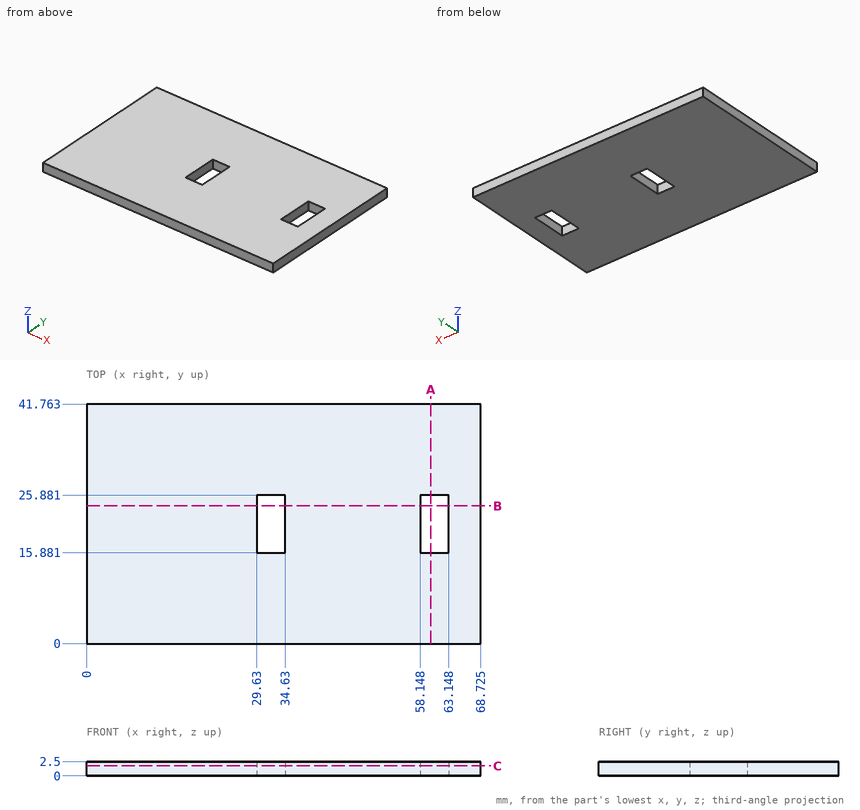
Job drawing, mm, ordinate dimensions from the low corner. One solid piece. Give positions to 0.01 mm unless a question says otherwise; leave off trailing zeros. Write each loop counter-clockwise with the first axis right and the second up, starting at its lowest first coordinate (ties: lowest second). Pieces come first, ordered by that corner, then holes. Notation, with made-up numbers: M -37.5,48.5 L -16.5,48.5 A21 ccw -16.5,67.5 Z; hole C 9,40.25 d3. An arc over 180 degrees is marked long. Put each result on its own line as item: value. Start each with the question number.
(1) Band-saw the part on C-C, the plane z = 1.75. Write the cut outline in (x, y) (1 decimal), and give its area (3 significant figures).
(2) Probe L1, parallel to Y at x = 34, z = 2.3; L2, parallel to X at y = 22.5, z = 0.7 (1 decimal). List the from-to ranges inside material, lowest first.
(3) Band-saw the part on A-A, the plane x = 60. Write the cut outline in (y, z).
(4) Band-saw the part on B-B, the plane y = 24. Write the cut outline in (x, z) (1 decimal), and give its area (3 significant figures).
Response values:
1. outline: M 0,0 L 68.7,0 L 68.7,41.8 L 0,41.8 Z; hole M 29.6,15.9 L 34.6,15.9 L 34.6,25.9 L 29.6,25.9 Z; hole M 58.1,15.9 L 63.1,15.9 L 63.1,25.9 L 58.1,25.9 Z
1. area: 2,770 mm2
2. L1: y = 0 to 15.88, 25.88 to 41.76
2. L2: x = 0 to 29.6, 34.6 to 58.1, 63.1 to 68.7
3. outline: M 0,0 L 15.88,0 L 15.88,2.5 L 0,2.5 Z; M 25.88,0 L 41.76,0 L 41.76,2.5 L 25.88,2.5 Z
4. outline: M 0,0 L 29.6,0 L 29.6,2.5 L 0,2.5 Z; M 34.6,0 L 58.1,0 L 58.1,2.5 L 34.6,2.5 Z; M 63.1,0 L 68.7,0 L 68.7,2.5 L 63.1,2.5 Z
4. area: 147 mm2
